```python
from build123d import *

# Parameters (mm, degrees)
SKETCH1_W                 = 146.05
SKETCH1_H                 = 85.725
BOSS_EXTRUDE1_DEPTH       = 3.175
F_6_CLEARANCE_HOLE1_D     = 4.3053
F_6_CLEARANCE_HOLE1_DEPTH = 12.7
F_6_CLEARANCE_HOLE1_TIP   = 1.293442612
SKETCH4_R                 = 6.35
SKETCH4_R_2               = 3.7703125
SKETCH4_R_3               = 1.190625
CUT_EXTRUDE1_DEPTH        = 4.175


with BuildPart() as part:
    # Sketch1 → Boss-Extrude1 (new body)
    with BuildSketch(Plane.XY):
        with Locations((-73.025, 42.8625)):
            Rectangle(SKETCH1_W, SKETCH1_H)
    extrude(amount=-BOSS_EXTRUDE1_DEPTH)

    # #6 Clearance Hole1
    with Locations(Plane(origin=(0, 0, -3.175), x_dir=(-1, 0, 0), z_dir=(0, 0, -1))):
        with Locations((4.8895, 71.4375), (53.34, 74.041), (92.075, 74.041), (141.1605, 71.4375), (109.982, 38.735), (141.1605, 14.2875), (33.528, 13.589), (4.8895, 14.2875)):
            Hole(F_6_CLEARANCE_HOLE1_D / 2, depth=F_6_CLEARANCE_HOLE1_DEPTH)
            with Locations((0, 0, -(F_6_CLEARANCE_HOLE1_DEPTH + F_6_CLEARANCE_HOLE1_TIP / 2))):  # 118° drill point
                Cone(0, F_6_CLEARANCE_HOLE1_D / 2, F_6_CLEARANCE_HOLE1_TIP, mode=Mode.SUBTRACT)

    # Sketch4 → Cut-Extrude1 (cut, through all)
    with BuildSketch(Plane(origin=(0, 0, -3.175), x_dir=(-1, 0, 0), z_dir=(0, 0, -1))):
        with Locations((20.828, 22.987)):
            Circle(SKETCH4_R)
        with Locations((123.19, 22.987)):
            Circle(SKETCH4_R)
        with Locations((33.782, 64.135)):
            Circle(SKETCH4_R_2)
        with Locations((72.39, 64.135)):
            Circle(SKETCH4_R_2)
        with Locations((110.998, 64.135)):
            Circle(SKETCH4_R_2)
        with Locations((91.694, 22.987)):
            Circle(SKETCH4_R_2)
        with Locations((53.086, 22.987)):
            Circle(SKETCH4_R_2)
        with Locations((37.582285256, 68.778041242)):
            Circle(SKETCH4_R_3)
        with Locations((76.190285256, 68.778041242)):
            Circle(SKETCH4_R_3)
        with Locations((114.798285256, 68.778041242)):
            Circle(SKETCH4_R_3)
        with Locations((56.886285256, 27.630041242)):
            Circle(SKETCH4_R_3)
        with Locations((95.494285256, 27.630041242)):
            Circle(SKETCH4_R_3)
    extrude(amount=-CUT_EXTRUDE1_DEPTH, mode=Mode.SUBTRACT)


solid = part.part
```
For this review, take the finished solid that the model builds, in its own axes (mm). Round coordinates to 2 decimals unless told otherwise and drop trailing zeros. Write each loop counter-clockwise with the first axis right and the second up, starting at its lowest first coordinate (ties: lowest second). Pieces come first, ordered by that corner, then holes. Notation, with made-up numbers: M -39.75,82.25 L -6.75,82.25 A15 ccw -6.75,111.25 Z; hole C -34.75,35.5 d6. An arc over 180 degrees is marked long. One line per item, written item: value. Start each with the question number.
(1) Insertion check: pin 1 (7 mm diameter, centred on x = -72.39, y = 64.135, fed in from +Z). The pin has a flat end and moves straight along its axis. Give the tip position at first contact, or say it passes through.
(2) We need section B-B (x = -53.34). Give the boundary of the cut face in (y, z) (3 decimals), and give its area (3 significant figures).
(3) Wall thickness on line 1 (X direction, y = 64, z = -2.1); line 2 (Y direction, x = -92, z = -2.05) (3 decimals); line 3 (X direction, y = 39, z = -1.4): over which ranges is each line inside the solid? List them lowest first.
(4) We need section C-C (z = -0.55). Count the separate pieces of the cut face and the enclosed holes in it, and give its area (3 significant figures).
(5) We need section A-A (x = -72.39). Give the boundary of the cut face in (y, z) (3 decimals), and give its area (3 significant figures).
(6) The part is to be moulded in two halves that separate along X. For faces 1 (the flat face through (0, 42, -2)), 2 (the cylindrical face through (-31.54, 12.76, -1.57)), 3 (the flat face through (-74, 0, -2)), say which applies: released by +X, released by -X, zero draft, split by the parting line, or undercut.
(7) We need section D-D (x = -123.19). Give the boundary of the cut face in (y, z) (3 decimals).
Result:
1. pin 1: through
2. outline: M 0,-3.175 L 19.225,-3.175 L 19.225,0 L 0,0 Z; M 26.749,-3.175 L 71.888,-3.175 L 71.888,0 L 26.749,0 Z; M 76.194,-3.175 L 85.725,-3.175 L 85.725,0 L 76.194,0 Z
2. area: 235 mm²
3. line 1: -146.05 to -114.77, -107.23 to -76.16, -68.62 to -37.55, -30.01 to 0
3. line 2: 0 to 19.229, 26.745 to 71.89, 76.192 to 85.725
3. line 3: -146.05 to -112.12, -107.85 to 0
4. separate pieces: 1
4. enclosed holes: 20
4. area: 11,900 mm²
5. outline: M 0,-3.175 L 60.365,-3.175 L 60.365,0 L 0,0 Z; M 67.905,-3.175 L 85.725,-3.175 L 85.725,0 L 67.905,0 Z
5. area: 248 mm²
6. face 1: released by +X
6. face 2: undercut
6. face 3: zero draft
7. outline: M 0,-3.175 L 16.637,-3.175 L 16.637,0 L 0,0 Z; M 29.337,-3.175 L 85.725,-3.175 L 85.725,0 L 29.337,0 Z
